Answer from the drawing. Dimensions are ordinates in mm from the lowest x, y and z of the part. Round coordinates to 2 decimals unless told otherwise and drop trailing zeros. Write each loop counter-clockwise with the first axis right and the second up, starting at its lowest first coordinate (ties: lowest second). Pieces come first, ordered by that corner, then holes. Notation, with made-up numbers: (-6, 85.5) -> (9, 85.5) arc R31 cw to (9, 115.5) -> close; hole circle Ø11 at (68.5, 21). An arc over 180 degrees is marked (long way). Answer as a JSON object with one key per item and string values. Group by question number.
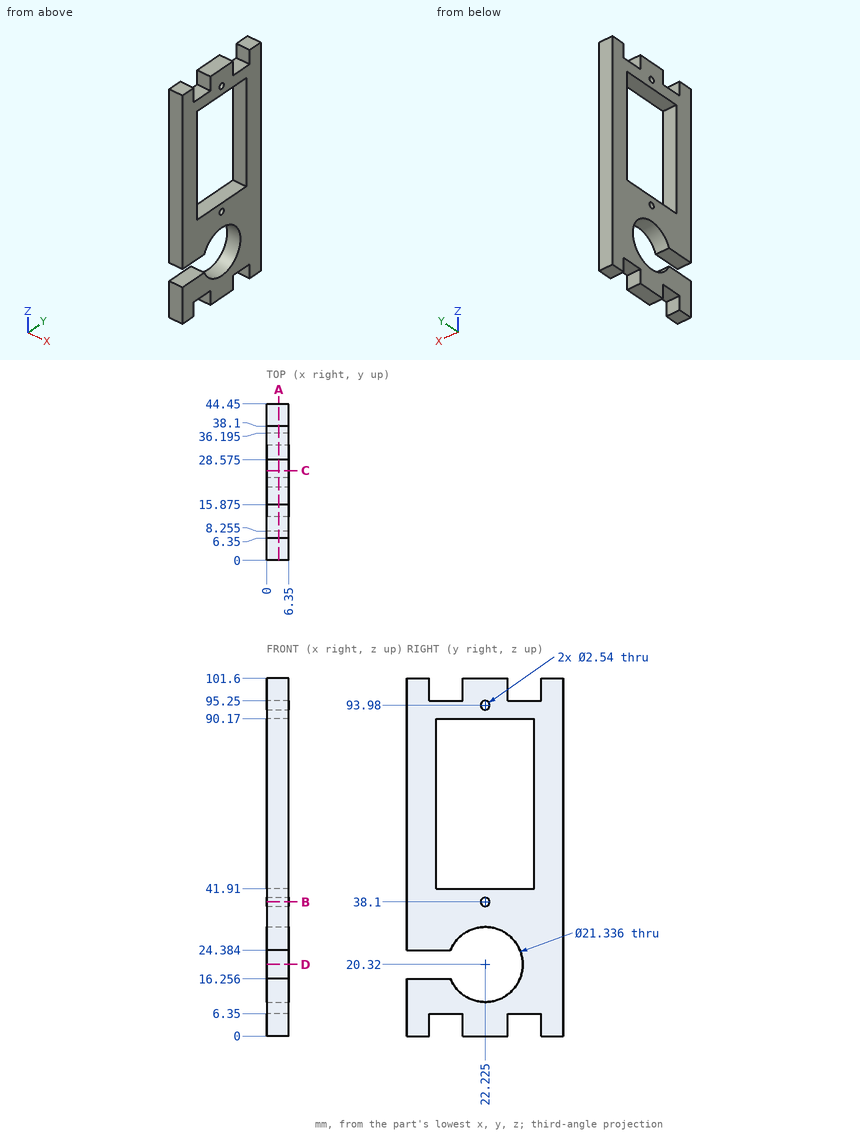
1) Straight lines are drawn through the part: L1, parallel to Y at x = 2.5, z = 4.5 (3 decimals); L2, parallel to Z at x = 0.5, y = 3.5; L3, parallel to Z at x = 2.75, y = 14. For each, find the intervals that lie inside material, in ascending order.
2) A cutting plane is placed at B-B on z = 38.1. Determine the outline of the cut face in (x, y) (3 decimals), plus the area to 3 significant figures.
3) A cutting plane is placed at D-D on z = 20.32. Determine the outline of the cut face in (x, y).
4) A cutting plane is placed at A-A on x = 3.5. State how many separate pieces and enclosed holes the cut face has, plus the area to 3 significant figures.
5) A cutting plane is placed at C-C on y = 25.5. Determine the outline of the cut face in (x, z), plus the area to 3 significant figures.
6) Each of these flat-tipped pins is pushed along its axis until it touches: P1, Ø1.9, axis at x = 4.5, z = 3, coming from the -Y side; P2, Ø1.5, axis at x = 1, y = 31.5, coming from the -Z side; P3, Ø2, axis at y = 22.225, z = 38.1, coming from the +X side. Where does it stop, or does it pass through?
Established:
{
 "1": {"L1": "y = 0 to 6.35, 15.875 to 28.575, 38.1 to 44.45", "L2": "z = 0 to 16.26, 24.38 to 101.6", "L3": "z = 6.35 to 13.53, 27.11 to 41.91, 90.17 to 95.25"},
 "2": {"outline": "(0, 0) -> (6.35, 0) -> (6.35, 20.955) -> (0, 20.955) -> close; (0, 23.495) -> (6.35, 23.495) -> (6.35, 44.45) -> (0, 44.45) -> close", "area": "266 mm²"},
 "3": {"outline": "(0, 32.89) -> (6.35, 32.89) -> (6.35, 44.45) -> (0, 44.45) -> close"},
 "4": {"separate pieces": "1", "enclosed holes": "3", "area": "2,460 mm²"},
 "5": {"outline": "(0, 0) -> (6.35, 0) -> (6.35, 10.17) -> (0, 10.17) -> close; (0, 30.47) -> (6.35, 30.47) -> (6.35, 41.91) -> (0, 41.91) -> close; (0, 90.17) -> (6.35, 90.17) -> (6.35, 101.6) -> (0, 101.6) -> close", "area": "210 mm²"},
 "6": {"P1": "stops at y = 0", "P2": "stops at z = 6.35", "P3": "passes through"}
}
